from build123d import *

# Parameters (mm, degrees)
SKETCH2_R           = 32.5
BOSS_EXTRUDE1_DEPTH = 10
SKETCH3_R           = 1.5
CUT_EXTRUDE2_DEPTH  = 48.037219306
CUT_EXTRUDE3_DEPTH  = 8
CUT_EXTRUDE5_START  = -5.5
CUT_EXTRUDE5_DEPTH  = 5.5
CIRPATTERN1_COUNT   = 3
CUT_EXTRUDE8_START  = -4.5
SKETCH8_R           = 22.4
CUT_EXTRUDE8_DEPTH  = 4.5
CHAMFER1_SIZE       = 4.429367468
CHAMFER1_SIZE_2     = 5
SKETCH7_R           = 6.1
CUT_EXTRUDE7_DEPTH  = 4
BOSS_EXTRUDE2_DEPTH = 4.5
SKETCH10_R          = 2.05
CUT_EXTRUDE9_DEPTH  = 7.5


with BuildPart() as part:
    # Sketch2 → Boss-Extrude1 (new body)
    with BuildSketch(Plane.XY):
        Circle(SKETCH2_R)
    extrude(amount=BOSS_EXTRUDE1_DEPTH)

    # Sketch3 → Cut-Extrude2 (cut, symmetric)
    with BuildSketch(Plane.XY):
        with Locations((0, 25)):
            Circle(SKETCH3_R)
    cut_extrude2 = extrude(amount=CUT_EXTRUDE2_DEPTH, both=True, mode=Mode.SUBTRACT)

    # Sketch4 → Cut-Extrude3 (cut)
    with BuildSketch(Plane.XY.offset(10)):
        Polygon((1.58771324, 22.25), (3.175426481, 25), (1.58771324, 27.75), (-1.58771324, 27.75), (-3.175426481, 25), (-1.58771324, 22.25), align=None)
    cut_extrude3 = extrude(amount=-CUT_EXTRUDE3_DEPTH, mode=Mode.SUBTRACT)

    # Sketch5 → Cut-Extrude5 (cut)
    with BuildSketch(Plane.XY.offset(10).offset(CUT_EXTRUDE5_START)):
        with BuildLine():
            Line((4.5, 25), (4.5, 32.186953879))
            ThreePointArc((4.5, 32.186953879), (0, 32.5), (-4.5, 32.186953879))
            Line((-4.5, 32.186953879), (-4.5, 25))
            ThreePointArc((-4.5, 25), (0, 20.5), (4.5, 25))
        make_face()
    cut_extrude5 = extrude(amount=CUT_EXTRUDE5_DEPTH, mode=Mode.SUBTRACT)

    # CirPattern1: Cut-Extrude2, Cut-Extrude3, Cut-Extrude5 ×3 about axis
    cirpattern1_axis = Axis((0, 0, 0), (0, 0, 1))
    add([cut_extrude2.rotate(cirpattern1_axis, i * 360 / CIRPATTERN1_COUNT) for i in range(1, CIRPATTERN1_COUNT)], mode=Mode.SUBTRACT)
    add([cut_extrude3.rotate(cirpattern1_axis, i * 360 / CIRPATTERN1_COUNT) for i in range(1, CIRPATTERN1_COUNT)], mode=Mode.SUBTRACT)
    add([cut_extrude5.rotate(cirpattern1_axis, i * 360 / CIRPATTERN1_COUNT) for i in range(1, CIRPATTERN1_COUNT)], mode=Mode.SUBTRACT)

    # Sketch8 → Cut-Extrude8 (cut)
    with BuildSketch(Plane.XY.offset(10).offset(CUT_EXTRUDE8_START)):
        with BuildLine():
            ThreePointArc((-30.12471973, -12.196362622), (-28.145825623, -16.25), (-25.62471973, -19.990591256))
            ThreePointArc((-25.62471973, -19.990591256), (0, -32.5), (25.62471973, -19.990591256))
            ThreePointArc((25.62471973, -19.990591256), (28.145825623, -16.25), (30.12471973, -12.196362622))
            ThreePointArc((30.12471973, -12.196362622), (28.145825623, 16.25), (4.5, 32.186953879))
            ThreePointArc((4.5, 32.186953879), (0, 32.5), (-4.5, 32.186953879))
            ThreePointArc((-4.5, 32.186953879), (-28.145825623, 16.25), (-30.12471973, -12.196362622))
        make_face()
        Circle(SKETCH8_R, mode=Mode.SUBTRACT)
    extrude(amount=CUT_EXTRUDE8_DEPTH, mode=Mode.SUBTRACT)

    # Chamfer1
    # the kernel refuses this chamfer: 5, 4.429367468 mm, written as the material it takes off along each edge
    with BuildSketch(Plane(origin=(-25.62471973, -19.990591256, 4.5), x_dir=(0.6702188271711587, -0.7421635424253312, 0), z_dir=(0, 0, 1)), Plane(origin=(30.12471973, -12.196362622, 4.5), x_dir=(0.3076230679174066, 0.9515083016375017, 0), z_dir=(0, 0, 1)), Plane(origin=(-4.5, 32.186953879, 4.5), x_dir=(-0.977841895088566, -0.2093447592121711, 0), z_dir=(0, 0, 1))) as chamfer1_piece_1:
        with BuildLine():
            Line((4.675763163, 0), (CHAMFER1_SIZE * 0.209344759198, CHAMFER1_SIZE * 0.977841895022))
            Line((CHAMFER1_SIZE * 0.209344759198, CHAMFER1_SIZE * 0.977841895022), (0, 0))
            ThreePointArc((0, 0), (2.403339666, -0.084130686), (4.675763163, 0))
        make_face()
    extrude(amount=13.02255857, mode=Mode.SUBTRACT)
    with BuildSketch(Plane(origin=(-30.12471973, -12.196362622, 4.5), x_dir=(-0.3141485775889788, 0.9493738311112337, 0), z_dir=(0, 0, 1)), Plane(origin=(25.62471973, -19.990591256, 4.5), x_dir=(-0.6651075666359972, -0.7467475643104184, 0), z_dir=(0, 0, 1)), Plane(origin=(4.5, 32.186953879, 4.5), x_dir=(0.9792561442249751, -0.20262626680081466, 0), z_dir=(0, 0, 1))) as chamfer1_piece_2:
        with BuildLine():
            Line((4.23053931, 0), (CHAMFER1_SIZE_2 * 0.202626266801, -CHAMFER1_SIZE_2 * 0.979256144225))
            Line((CHAMFER1_SIZE_2 * 0.202626266801, -CHAMFER1_SIZE_2 * 0.979256144225), (0, 0))
            ThreePointArc((0, 0), (2.170160838, 0.068863095), (4.23053931, 0))
        make_face()
    extrude(amount=13.85841494, mode=Mode.SUBTRACT)

    # Sketch7 → Cut-Extrude7 (cut)
    with BuildSketch(Plane(origin=(0, 0, 0), x_dir=(-1, 0, 0), z_dir=(0, 0, -1))):
        Circle(SKETCH7_R)
    extrude(amount=-CUT_EXTRUDE7_DEPTH, mode=Mode.SUBTRACT)

    # Sketch9 → Boss-Extrude2 (add)
    with BuildSketch(Plane.XY.offset(10)):
        with BuildLine():
            ThreePointArc((-3.466157521, 22.1302), (0, 20.5), (3.466157521, 22.1302))
            ThreePointArc((3.466157521, 22.1302), (19.398969045, 11.2), (20.898394151, -8.063319533))
            ThreePointArc((20.898394151, -8.063319533), (17.753520778, -10.25), (17.43223663, -14.066880467))
            ThreePointArc((17.43223663, -14.066880467), (0, -22.4), (-17.43223663, -14.066880467))
            ThreePointArc((-17.43223663, -14.066880467), (-17.753520778, -10.25), (-20.898394151, -8.063319533))
            ThreePointArc((-20.898394151, -8.063319533), (-19.398969045, 11.2), (-3.466157521, 22.1302))
        make_face()
    extrude(amount=BOSS_EXTRUDE2_DEPTH)

    # Sketch10 → Cut-Extrude9 (cut)
    with BuildSketch(Plane.XY.offset(14.5)):
        with Locations((-8.645741201, -15.215162144)):
            Circle(SKETCH10_R)
        with Locations((-17.49958754, -0.120149557)):
            Circle(SKETCH10_R)
        with Locations((-8.853846339, 15.095012587)):
            Circle(SKETCH10_R)
        with Locations((8.645741201, 15.215162144)):
            Circle(SKETCH10_R)
        with Locations((17.49958754, 0.120149557)):
            Circle(SKETCH10_R)
        with Locations((8.853846339, -15.095012587)):
            Circle(SKETCH10_R)
    extrude(amount=-CUT_EXTRUDE9_DEPTH, mode=Mode.SUBTRACT)


solid = part.part
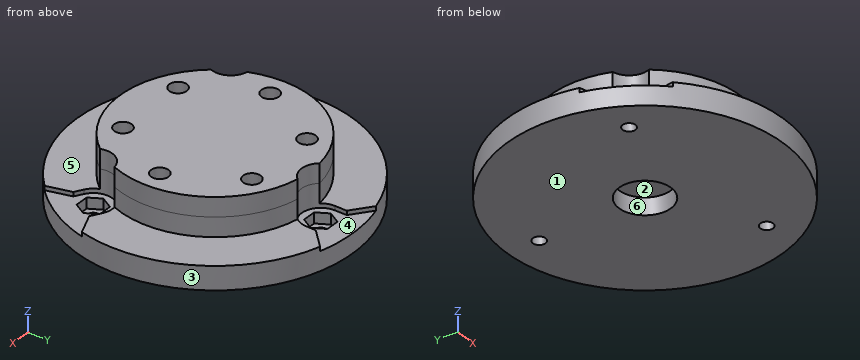
Geometry check sheet. Reference: the model listing, model coordinates, mm. Face numbers are marked on the shaded views. A direction names the side the tool comes from. Coordinates: 2 decimals unless noted, no trailing zeros. Order: outer loops, then holes, each group sorted by start corner. A loop starts at its lowest first (then second) coordinate and runs counter-clockwise, first axis right, second up. Notation, with made-up numbers: (77, 68.25) -> (128, 68.25) arc R29 cw to (128, 103.25) -> close; hole circle Ø8 at (-15, 2). An arc over 180 degrees is marked (long way). Use a Markdown table: item, result. Add a question column.
1. Go/stop test with flat-tipped pins: pin 1 Ø15.5 at (x, y) = (-25, -17) entering from +Z; pin 2 Ø4.5 at (x, y) = (20.5, -12.5) entering from +Z; pin 3 Ø1.2 at (x, z) = (-21, 2.5) entering from -Y. Record where each tip stops, or that it passes through.
2. Set-up check for the marked faces 4, 5 and 6: record each of +Z, -Z, +X, -X, +Y, -Y from which the full face is reachable in a straight line by a thin tool's end or side.
3. Cross-section at A-A (z = 8.5). Enter the section's corners in (x, y), and give its area (3 significant figures).
4. Cross-section at B-B (y = -3.5). Enter the section's corners in (x, z), and give its area (3 significant figures).
5. Cross-section at C-C (x = -12.5). Enter the section's corners in (y, z), and give its area (3 significant figures).
6. Mould release check, pull along Y, two halves, no side actions. Record for the marked faces 1, 2 and 3: pulls with the +Y half, pulls with the -Y half, needs draft (parallel to the pull), parting line crosses it, or undercut.
7. Cross-section at D-D (y = -27.5). Enter the section's corners in (x, z), and give its area (3 significant figures).
8. Material ranges on L1, parallel to Y at x = 0, z = 1; L2, parallel to Y at x = -1, z = 3.25; L3, parallel to X at y = -11, z = 3.25, recorded low to high.
Filled sheet:
| question | item | result |
|---|---|---|
| 1 | pin 1 | z = 5.5 |
| 1 | pin 2 | z = 4.5 |
| 1 | pin 3 | y = -25.3 |
| 2 | face 4 | +Z, +Y |
| 2 | face 5 | +Z, -Y |
| 2 | face 6 | -Z |
| 3 | outline | (-20.9, -8.06) arc R4.5 cw to (-17.43, -14.07) arc R22.4 ccw to (17.43, -14.07) arc R4.5 cw to (20.9, -8.06) arc R22.4 ccw to (3.47, 22.13) arc R4.5 cw to (-3.47, 22.13) arc R22.4 ccw to start; hole circle Ø4.1 at (-17.5, -0.12); hole circle Ø4.1 at (-8.85, 15.1); hole circle Ø4.1 at (-8.65, -15.22); hole circle Ø4.1 at (8.65, 15.22); hole circle Ø4.1 at (8.85, -15.1); hole circle Ø4.1 at (17.5, 0.12) |
| 3 | area | 1,470 mm2 |
| 4 | outline | (-32.31, 0) -> (-5, 0) -> (-5, 4) -> (5, 4) -> (5, 0) -> (32.31, 0) -> (32.31, 5.5) -> (22.12, 5.5) -> (22.12, 14.5) -> (-22.12, 14.5) -> (-22.12, 5.5) -> (-32.31, 5.5) -> close |
| 4 | area | 714 mm2 |
| 5 | outline | (-30, 0) -> (30, 0) -> (30, 5.5) -> (18.59, 5.5) -> (18.59, 14.5) -> (-18.59, 14.5) -> (-18.59, 5.5) -> (-30, 5.5) -> close |
| 5 | area | 665 mm2 |
| 6 | face 1 | needs draft |
| 6 | face 2 | undercut |
| 6 | face 3 | parting line crosses it |
| 7 | outline | (-17.32, 0) -> (17.32, 0) -> (17.32, 5.5) -> (-17.32, 5.5) -> close |
| 7 | area | 191 mm2 |
| 8 | L1 | -32.5 to -6.1, 6.1 to 23.5, 26.5 to 32.5 |
| 8 | L2 | -32.48 to -6.02, 6.02 to 22.25, 27.75 to 32.48 |
| 8 | L3 | -30.58 to -23.96, -19.34 to 19.34, 23.96 to 30.58 |
